For this review, take the finished solid that the model builds, in its own axes (mm). A direction names the side the tool comes from. Give positions to 0.01 mm unless a question says otherwise; leave off trailing zeros. Write each loop counter-clockwise with the first axis right and the second up, starting at its lowest first coordinate (ties: lowest second). Pieces come first, ordered by that corner, then holes. Notation, with made-up numbers: M 8.5,2.5 L 50.5,2.5 A31 ccw 50.5,36.5 Z; hole C 78,-40 d6. An arc over 180 degrees is marked long. One line per item, written item: value. Start each with the question number.
Item 1: Consider section C-C, the plane z = 13.5. Write out the cut boundary in (x, y), and give its area (3 significant figures).
Item 2: Consider section D-D, the plane y = 4.75. Write out the cut boundary in (x, z), and give its area (3 significant figures).
Item 3: Mouldability with a two-part tool opening along X and no side actions: class faces 1 (the face through (3, 9, 29)), 2 (the face through (6.396, 5.426, 28.014)), 3 (the face through (7, 10, 28)) as released by +X, released by -X, zero draft, split by the parting line, or undercut.
Item 4: Tool access review of faces 4 (the face through (-43, 18.5, 28)), 5 (the face through (-43, 10, 29)), 6 (the face through (3, 18.5, 28)): name each direction out of +Z, -Z, +X, -X, +Y, -Y from which nothing blocks a thin tool from reaching the whole face with its end or side.
Item 5: To check wall thickness, follow probe 1 along Y at (x, z) = (4.25, 27.7); probe 2 along Z at (x, y) = (-39, 17.25); probe 3 along X at (y, z) = (6.5, 20). State the ranges of each line that lie inside material, in increasing order.
Item 6: Consider section B-B, the plane x = -19. Write out the cut boundary in (y, z), and give its area (3 significant figures).
Item 7: Clearance check with flat-ended pins moving along their axes: pin 1 Ø2 at (x, z) = (4, 27.5) entering from -Y; pin 2 Ø5 at (x, y) = (4.25, 4.75) entering from +Z; pin 3 Ø2 at (y, z) = (6.5, 36.5) entering from +X. State where each tip first meets the part, or that it passes through.
Item 8: Consider section A-A, the plane y = 13. Write out the cut boundary in (x, z), and give its area (3 significant figures).
Autodesk Inventor part; units mm, degrees
ref_plane "YZ Plane" through (0, 0, 0) normal (1, 0, 0) x (0, 1, 0)
ref_plane "XZ Plane" through (0, 0, 0) normal (0, 1, 0) x (-1, 0, 0)
ref_plane "XY Plane" through (0, 0, 0) normal (0, 0, 1) x (1, 0, 0)
sketch "Skizze1" plane through (0, 0, 0) normal (0, 0, 1) x (1, 0, 0)
  line L0 (0, 0) -> (-40, 0)
  line L1 (-40, 0) -> (-40, 19)
  line L2 (-40, 19) -> (0, 19)
  line L3 (0, 19) -> (0, 0)
  dimension "d0" = 40
  dimension "d1" = 19
extrude "Extrusion1" add sketch "Skizze1" along normal blind 35
sketch "Skizze2" plane through (0, 0, 35) normal (0, 0, 1) x (1, 0, 0)
  line L0 (-40, 19) -> (0, 19)
  circle A0 centre (-30, 9.5) radius 9.5
  dimension "d4" = 10
extrude "Extrusion2" add sketch "Skizze2" along normal blind 2
sketch "Skizze3" plane through (0, 0, 35) normal (0, 0, 1) x (1, 0, 0)
  line L0 (0, 19) -> (0, 0)
  line L1 (-37, 3.6605) -> (-37, 17.3389)
  line L2 (-7, 1) -> (-7, 18)
  line L3 (-7, 18) -> (-30, 18)
  line L4 (-30, 18) -> (-30, 1)
  line L5 (-30, 1) -> (-7, 1)
  dimension "d13" = 17
extrude "Extrusion3" add sketch "Skizze3" along normal blind 2
sketch "Skizze4" plane through (0, 0, 37) normal (0, 0, 1) x (1, 0, 0)
  arc A0 (-25.7574, 18) -> (-25.7574, 1) centre (-30, 9.5) ccw
  circle A1 centre (-30, 9.5) radius 6
  point P0 (0, 0)
  dimension "d16" = 12
extrude "Extrusion4" add sketch "Skizze4" along normal blind 2
sketch "Skizze6" plane through (-40, 0, 0) normal (-1, 0, 0) x (0, 0, 1)
  line L0 (27, 18.5) -> (29, 18.5)
  line L1 (29, 18.5) -> (29, 0.5)
  line L2 (29, 0.5) -> (27, 0.5)
  line L3 (27, 0.5) -> (27, 18.5)
  dimension "d23" = 2
  dimension "d24" = 18
extrude "Extrusion5" add sketch "Skizze6" along normal blind 7
sketch "Skizze7" plane through (-40, 0.5, 29) normal (0, 0, 1) x (1, 0, 0)
  circle A0 centre (-4.25, 4.25) radius 2.25
  circle A1 centre (-4.25, 13.75) radius 2.25
  point P0 (40, -0.5)
  dimension "d27" = 4.5
  dimension "d28" = 4.5
extrude "Extrusion6" cut sketch "Skizze7" against normal blind 2 contours A0
sketch "Skizze8" plane through (-40, 0.5, 29) normal (0, 0, 1) x (1, 0, 0)
  circle A0 centre (-4.25, 13.75) radius 2.25
  point P0 (40, -0.5)
  dimension "d31" = 4.5
extrude "Extrusion7" cut sketch "Skizze8" against normal blind 2
fillet "Rundung1" radius 1 1 edges at (-47, 0.5, 28)
fillet "Rundung2" radius 1 1 edges at (-47, 18.5, 28)
sketch "Skizze9" plane through (0, 0, 0) normal (1, 0, 0) x (0, 0, -1)
  line L0 (-27, 0.5) -> (-29, 0.5)
  line L1 (-29, 0.5) -> (-29, 18.5)
  line L2 (-29, 18.5) -> (-27, 18.5)
  line L3 (-27, 18.5) -> (-27, 0.5)
  dimension "d36" = 2
  dimension "d37" = 18
extrude "Extrusion8" add sketch "Skizze9" along normal blind 7
sketch "Skizze10" plane through (0, 0.5, 29) normal (0, 0, 1) x (1, 0, 0)
  circle A0 centre (4.25, 4.25) radius 2.25
  point P0 (0, -0.5)
  dimension "d40" = 4.5
extrude "Extrusion9" cut sketch "Skizze10" against normal blind 2
sketch "Skizze11" plane through (0, 0.5, 29) normal (0, 0, 1) x (1, 0, 0)
  circle A0 centre (4.25, 13.75) radius 2.25
  point P0 (0, -0.5)
  dimension "d43" = 4.5
extrude "Extrusion10" cut sketch "Skizze11" against normal blind 2
fillet "Rundung3" radius 1 1 edges at (7, 18.5, 28)
fillet "Rundung4" radius 1 1 edges at (7, 0.5, 28)
properties part number "servo" material "PC/ABS-Kunststoff"
Model answer:
1. outline: M -40,0 L 0,0 L 0,19 L -40,19 Z
1. area: 760 mm2
2. outline: M -47,27 L -46.5,27 L -46.5,29 L -47,29 Z; M -42,27 L -40,27 L -40,0 L 0,0 L 0,27 L 2,27 L 2,29 L 0,29 L 0,35 L -7,35 L -7,37 L -26.33,37 L -26.33,39 L -33.67,39 L -33.67,37 L -38.23,37 L -38.23,35 L -40,35 L -40,29 L -42,29 Z; M 6.5,27 L 7,27 L 7,29 L 6.5,29 Z
2. area: 1,490 mm2
3. face 1: zero draft
3. face 2: undercut
3. face 3: released by +X
4. face 4: +Z, -Z, -X, +Y
4. face 5: +Z, -X, +Y, -Y
4. face 6: +Z, -Z, +X, +Y
5. probe 1: y = 0.5 to 2.5, 7 to 12, 16.5 to 18.5
5. probe 2: z = 0 to 35
5. probe 3: x = -40 to 0
6. outline: M 0,0 L 19,0 L 19,35 L 18,35 L 18,37 L 1,37 L 1,35 L 0,35 Z
6. area: 699 mm2
7. pin 1: stops at y = 0.5
7. pin 2: stops at z = 29
7. pin 3: stops at x = -7
8. outline: M -47,27 L -46.12,27 L -46.12,29 L -47,29 Z; M -42.38,27 L -40,27 L -40,0 L 0,0 L 0,27 L 2.38,27 L 2.38,29 L 0,29 L 0,35 L -7,35 L -7,37 L -25.13,37 L -25.13,39 L -34.87,39 L -34.87,37 L -38.83,37 L -38.83,35 L -40,35 L -40,29 L -42.38,29 Z; M 6.12,27 L 7,27 L 7,29 L 6.12,29 Z
8. area: 1,500 mm2
